Read the model definition and answer for the solid it produces. Units are mm, in the model's axes. A direction names the side the tool comes from. Give positions to 0.01 mm unless a question says otherwise; leave off trailing zeros. Order: outer loops, then holes, each group sorted by start corner. A loop starts at its lowest first (then second) coordinate and runs counter-clockwise, first axis right, second up. Notation, with made-up numbers: M -19,-6.5 L -12,-6.5 A23 ccw -12,20.5 Z; hole C 62.5,72 d4. An arc over 180 degrees is marked long. One line per item, written item: value. Start each with the question number.
from build123d import *

# Parameters (mm, degrees)
ESQUISSE1_R        = 15
ESQUISSE1_R_2      = 13.35
BOSS_EXTRU_1_DEPTH = 21
BOSS_EXTRU_2_START = 1
ESQUISSE2_R        = 15.2
ESQUISSE2_R_2      = 13.35
BOSS_EXTRU_2_DEPTH = 1
ESQUISSE3_R        = 15
ESQUISSE3_R_2      = 7.7
ESQUISSE3_R_3      = 1.5
BOSS_EXTRU_3_DEPTH = 1.5


with BuildPart() as part:
    # Esquisse1 → Boss.-Extru.1 (new body)
    with BuildSketch(Plane.XY):
        with Locations(Location((0, 0, 0), (0, 0, 180))):
            Circle(ESQUISSE1_R)
        with Locations(Location((0, 0, 0), (0, 0, 180))):
            Circle(ESQUISSE1_R_2, mode=Mode.SUBTRACT)
    extrude(amount=BOSS_EXTRU_1_DEPTH)

    # Esquisse2 → Boss.-Extru.2 (add)
    with BuildSketch(Plane(origin=(0, 0, 0), x_dir=(-1, 0, 0), z_dir=(0, 0, -1)).offset(BOSS_EXTRU_2_START)):
        Circle(ESQUISSE2_R)
        Circle(ESQUISSE2_R_2, mode=Mode.SUBTRACT)
    extrude(amount=-BOSS_EXTRU_2_DEPTH)

    # Esquisse3 → Boss.-Extru.3 (add)
    with BuildSketch(Plane.XY.offset(21)):
        with Locations(Location((0, 0, 0), (0, 0, 180))):
            Circle(ESQUISSE3_R)
        Circle(ESQUISSE3_R_2, mode=Mode.SUBTRACT)
        with Locations((0, -10)):
            Circle(ESQUISSE3_R_3, mode=Mode.SUBTRACT)
        with Locations((0, 10)):
            Circle(ESQUISSE3_R_3, mode=Mode.SUBTRACT)
        with Locations((-10, 0)):
            Circle(ESQUISSE3_R_3, mode=Mode.SUBTRACT)
        with Locations((10, 0)):
            Circle(ESQUISSE3_R_3, mode=Mode.SUBTRACT)
    extrude(amount=BOSS_EXTRU_3_DEPTH)


solid = part.part
Q1. Each of these flat-tipped pins is pushed along its axis until it touches: pin 1 (3 mm diameter, centred on y = 4, z = 3.5, fed in from +X); pin 2 (4 mm diameter, centred on x = 0, y = -10, fed in from -Z); pin 3 (8 mm diameter, centred on x = 4.5, z = 17.5, fed in from +Y); pin 4 (16 mm diameter, centred on x = 0, y = 0, fed in from +Z). Where does it stop, or does it pass through?
Q2. Find section A-A, the plane x = 0. Give the vertices of the cut face in (y, z), then the cut area to 3 significant figures.
Q3. Consider probe 1 along Y at (x, z) = (0, 5.75); probe 2 along Y at (x, z) = (0, 21.4); probe 3 along Y at (x, z) = (0, -0.8). Determine where each line is inside the solid, lowest interval first.
Q4. A tool of negligible diameter and unlimited length cuts with its end or side. For faces 1 (the flat face through (-6, 6, 21)), 2 (the cylindrical face through (8.5, 0.07, 21.74)), from which of +Z, -Z, +X, -X, +Y, -Y can it reach the whole face along a straight path? Write none if from no direction.
Q5. Determine the mould class of faces 3 (the cylindrical face through (-8.06, -12.65, 11.09)), 4 (the flat face through (4, -7, 22.5)), 5 (the cylindrical face through (-1.669, -7.517, 21.74)) for opening direction Y: released by +Y, released by -Y, zero draft, split by the parting line, or undercut.
Q6. Find section C-C, the plane x = -10. Give the vertices of the cut face in (y, z).
Evaluation:
1. pin 1: x = 14.79
1. pin 2: z = 21
1. pin 3: y = 14.99
1. pin 4: z = 22.5
2. outline: M -15.2,-1 L -13.35,-1 L -13.35,21 L -11.5,21 L -11.5,22.5 L -15,22.5 L -15,0 L -15.2,0 Z; M -8.5,21 L -7.7,21 L -7.7,22.5 L -8.5,22.5 Z; M 7.7,21 L 8.5,21 L 8.5,22.5 L 7.7,22.5 Z; M 11.5,21 L 13.35,21 L 13.35,-1 L 15.2,-1 L 15.2,0 L 15,0 L 15,22.5 L 11.5,22.5 Z
2. area: 85.9 mm2
3. probe 1: -15 to -13.35, 13.35 to 15
3. probe 2: -15 to -11.5, -8.5 to -7.7, 7.7 to 8.5, 11.5 to 15
3. probe 3: -15.2 to -13.35, 13.35 to 15.2
4. face 1: -Z
4. face 2: +Z, -Z
5. face 3: split by the parting line
5. face 4: zero draft
5. face 5: undercut
6. outline: M -11.45,-1 L -8.84,-1 L -8.84,21 L -1.5,21 L -1.5,22.5 L -11.18,22.5 L -11.18,0 L -11.45,0 Z; M 1.5,21 L 8.84,21 L 8.84,-1 L 11.45,-1 L 11.45,0 L 11.18,0 L 11.18,22.5 L 1.5,22.5 Z
